```python
from build123d import *

# Parameters (mm, degrees)
SKETCH1_W           = 20
SKETCH1_H           = 45
BOSS_EXTRUDE1_DEPTH = 30
SKETCH2_W           = 40
SKETCH2_H           = 40
BOSS_EXTRUDE2_DEPTH = 20
FILLET1_R           = 10


with BuildPart() as part:
    # Sketch1 → Boss-Extrude1 (new body)
    with BuildSketch(Plane.XY):
        with Locations((-20, -22.5)):
            Rectangle(SKETCH1_W, SKETCH1_H)
    extrude(amount=BOSS_EXTRUDE1_DEPTH)

    # Sketch2 → Boss-Extrude2 (add)
    with BuildSketch(Plane.XY):
        with Locations((-10, -25)):
            Rectangle(SKETCH2_W, SKETCH2_H)
    extrude(amount=-BOSS_EXTRUDE2_DEPTH)

    # Fillet1
    fillet1_edges = [part.edges().sort_by_distance(p)[0] for p in [
        (10, -5, -10),
        (-20, 0, 30),
    ]]
    fillet(fillet1_edges, radius=FILLET1_R)


solid = part.part
```
Geometry check sheet. Reference: the model listing, model coordinates, mm. A direction names the side the tool comes from. Round coordinates to 2 decimals unless told otherwise and drop trailing zeros. Order: outer loops, then holes, each group sorted by start corner. A loop starts at its lowest first (then second) coordinate and runs counter-clockwise, first axis right, second up. Notation, with made-up numbers: (68, 1) - (103, 1) arc R25 cw to (103, 20) - close; hole circle Ø4 at (34.25, 44). An arc over 180 degrees is marked (long way). Use a Markdown table: item, result. Add a question column.
(1) Sectioned sample at D-D, the plane y = -13. Enter the section's corners in (x, z).
(2) Sectioned sample at C-C, the plane y = -7.5. Enter the section's corners in (x, z).
(3) Sectioned sample at B-B, the plane z = -8. Enter the section's corners in (x, y).
(4) Material ranges on line 1 along Z through (x, y) = (-6.5, -38.5); line 2 along Y through (x, z) = (-25.5, -10); line 3 along X through (y, z) = (-37.5, 10.5), recorded low to high. Write a range as [from, to].
(5) Depth check by flat-ended pin: pin 1 (10 mm diameter, centred on x = 0.5, y = -31, fed in from +Z); pin 2 (1 mm diameter, centred on y = -18, z = 22.5, fed in from +X); pin 3 (16 mm diameter, centred on x = -9.5, z = -13, fed in from +Y). Enter the tip coordinate at first touch or a pass-through.
(6) Sectioned sample at A-A, the plane x = -26. Enter the section's corners in (y, z), and give its area (3 significant figures).
(7) Tool access check on faces 1 (the flat face through (-30, -23, 5)), 2 (the flat face through (-10, -23, 15)), 3 (the flat face through (-15, -5, -10)). Record the directions out of +Z, -Z, +X, -X, +Y, -Y that give a thin tool (end or side, any length) a straight path to the whole face; none if there is none.
Answers below:
| question | item | result |
|---|---|---|
| 1 | outline | (-30, -20) - (9.8, -20) - (9.8, 0) - (-10, 0) - (-10, 30) - (-30, 30) - close |
| 2 | outline | (-30, -20) - (6.61, -20) - (6.61, 0) - (-10, 0) - (-10, 29.68) - (-30, 29.68) - close |
| 3 | outline | (-30, -45) - (10, -45) - (10, -15) arc R10 ccw to (0, -5) - (-30, -5) - close |
| 4 | line 1 | [-20, 0] |
| 4 | line 2 | [-45, -5] |
| 4 | line 3 | [-30, -10] |
| 5 | pin 1 | z = 0 |
| 5 | pin 2 | x = -10 |
| 5 | pin 3 | y = -5 |
| 6 | outline | (-45, -20) - (-5, -20) - (-5, 0) - (0, 0) - (0, 20) arc R10 ccw to (-10, 30) - (-45, 30) - close |
| 6 | area | 2,130 mm² |
| 7 | face 1 | +Z, -Z, -X, +Y, -Y |
| 7 | face 2 | +Z, +X, +Y, -Y |
| 7 | face 3 | -Z, +X, -X, +Y |
